from build123d import *

# Parameters (mm, degrees)
F0_R     = 4.1275
F0_R_2   = 4.0005
F0_W     = 107.95
F0_H     = 76.2
F0_R_3   = 3.429
F0_W_2   = 712.238387
F0_H_2   = 25.4
F0_W_3   = 19.05
F0_H_3   = 50.8
F1_DEPTH = 1.5748
F2_W     = 19.05
F2_H     = 1.5748
F3_DEPTH = 25.4


with BuildPart() as f1:
    # F0 (on Front) → F1 (new body)
    with BuildSketch(Plane.XZ):
        with BuildLine():
            Line((0, 71.12), (0, 0))
            Line((0, 0), (152.4, 0))
            Line((152.4, 0), (864.638387, 0))
            ThreePointArc((864.638387, 0), (866.755792, 0.026154), (868.871905, 0.1046))
            ThreePointArc((868.871905, 0.1046), (878.359069, 1.105153), (887.676316, 3.15364))
            ThreePointArc((887.676316, 3.15364), (903.696678, 9.414938), (918.144584, 18.748418))
            ThreePointArc((918.144584, 18.748418), (921.788387, 21.829358), (925.255116, 25.108271))
            Line((925.255116, 25.108271), (873.880221, 76.483166))
            ThreePointArc((873.880221, 76.483166), (871.544457, 74.285755), (868.777424, 72.664665))
            Line((868.777424, 72.664665), (830.221387, 55.5625))
            Line((830.221387, 55.5625), (830.221387, 36.5125))
            Line((830.221387, 36.5125), (747.671387, 36.5125))
            Line((747.671387, 36.5125), (747.671387, 112.7125))
            Line((747.671387, 112.7125), (830.221387, 112.7125))
            Line((830.221387, 112.7125), (830.221387, 100.0125))
            Line((830.221387, 100.0125), (862.984297, 100.0125))
            ThreePointArc((862.984297, 100.0125), (868.988044, 98.689863), (873.880221, 94.966834))
            Line((873.880221, 94.966834), (925.255116, 146.341729))
            ThreePointArc((925.255116, 146.341729), (921.788387, 149.620642), (918.144584, 152.701582))
            ThreePointArc((918.144584, 152.701582), (901.799905, 162.976519), (883.570429, 169.333333))
            ThreePointArc((883.570429, 169.333333), (874.163387, 170.91919), (864.638387, 171.45))
            Line((864.638387, 171.45), (858.288387, 171.45))
            Line((858.288387, 171.45), (839.238387, 171.45))
            Line((839.238387, 171.45), (839.238387, 222.25))
            Line((839.238387, 222.25), (839.238387, 273.05))
            Line((839.238387, 273.05), (839.238387, 323.85))
            Line((839.238387, 323.85), (595.3125, 200.025))
            Line((595.3125, 200.025), (455.231453, 200.025))
            Line((455.231453, 200.025), (439.727616, 200.025))
            Line((439.727616, 200.025), (356.5525, 200.025))
            Line((356.5525, 200.025), (356.5525, 151.765))
            Line((356.5525, 151.765), (303.2125, 151.765))
            Line((303.2125, 151.765), (303.2125, 200.025))
            Line((303.2125, 200.025), (71.490397, 200.025))
            Line((71.490397, 200.025), (0, 158.75))
            Line((0, 158.75), (0, 106.045))
            Line((0, 106.045), (138.1125, 106.045))
            ThreePointArc((138.1125, 106.045), (155.575, 88.5825), (138.1125, 71.12))
            Line((138.1125, 71.12), (0, 71.12))
        make_face()
        with Locations((184.0865, 65.0875)):
            Circle(F0_R, mode=Mode.SUBTRACT)
        Polygon((206.375, 41.91), (206.375, 88.5825), (206.375, 111.76), (266.7, 111.76), (266.7, 41.91), align=None, mode=Mode.SUBTRACT)
        with Locations((31.0642, 136.9695)):
            Circle(F0_R_2, mode=Mode.SUBTRACT)
        with Locations((184.0865, 109.8169)):
            Circle(F0_R, mode=Mode.SUBTRACT)
        with Locations((227.838, 136.9695)):
            Circle(F0_R_2, mode=Mode.SUBTRACT)
        with Locations((424.6118, 136.9695)):
            Circle(F0_R_2, mode=Mode.SUBTRACT)
        with BuildLine():
            ThreePointArc((853.652887, 31.8135), (848.509387, 36.957), (853.652887, 42.1005))
            Line((853.652887, 42.1005), (863.939887, 42.1005))
            ThreePointArc((863.939887, 42.1005), (867.576891, 40.594004), (869.083387, 36.957))
            ThreePointArc((869.083387, 36.957), (867.576891, 33.319996), (863.939887, 31.8135))
            Line((863.939887, 31.8135), (853.652887, 31.8135))
        make_face(mode=Mode.SUBTRACT)
        with Locations((642.388387, 74.6252)):
            Rectangle(F0_W, F0_H, mode=Mode.SUBTRACT)
        with BuildLine():
            ThreePointArc((715.794387, 106.0577), (719.921887, 110.1852), (724.049387, 106.0577))
            Line((724.049387, 106.0577), (724.049387, 47.6377))
            ThreePointArc((724.049387, 47.6377), (719.921887, 43.5102), (715.794387, 47.6377))
            Line((715.794387, 47.6377), (715.794387, 106.0577))
        make_face(mode=Mode.SUBTRACT)
        with Locations((621.3856, 136.9695)):
            Circle(F0_R_2, mode=Mode.SUBTRACT)
        with Locations((816.314887, 137.033)):
            Circle(F0_R_2, mode=Mode.SUBTRACT)
        with BuildLine():
            ThreePointArc((853.652887, 129.2225), (848.509387, 134.366), (853.652887, 139.5095))
            Line((853.652887, 139.5095), (863.939887, 139.5095))
            ThreePointArc((863.939887, 139.5095), (867.576891, 138.003004), (869.083387, 134.366))
            ThreePointArc((869.083387, 134.366), (867.576891, 130.728996), (863.939887, 129.2225))
            Line((863.939887, 129.2225), (853.652887, 129.2225))
        make_face(mode=Mode.SUBTRACT)
        with BuildLine():
            ThreePointArc((244.6655, 177.038), (247.988195, 175.661695), (249.3645, 172.339))
            ThreePointArc((249.3645, 172.339), (247.988195, 169.016305), (244.6655, 167.64))
            Line((244.6655, 167.64), (235.2675, 167.64))
            ThreePointArc((235.2675, 167.64), (230.5685, 172.339), (235.2675, 177.038))
            Line((235.2675, 177.038), (244.6655, 177.038))
        make_face(mode=Mode.SUBTRACT)
        with Locations((371.7925, 190.119)):
            Circle(F0_R_3, mode=Mode.SUBTRACT)
        with Locations((757.513887, 160.655)):
            Circle(F0_R_2, mode=Mode.SUBTRACT)
        with Locations((807.577287, 160.655)):
            Circle(F0_R_2, mode=Mode.SUBTRACT)
        with BuildLine():
            ThreePointArc((873.880221, 94.966834), (876.39713, 90.647253), (877.271797, 85.725))
            Line((877.271797, 85.725), (950.363387, 85.725))
            ThreePointArc((950.363387, 85.725), (950.230582, 90.49489), (949.832577, 95.25))
            ThreePointArc((949.832577, 95.25), (943.83796, 118.530537), (931.614968, 139.231197))
            ThreePointArc((931.614968, 139.231197), (928.534029, 142.875), (925.255116, 146.341729))
            Line((925.255116, 146.341729), (873.880221, 94.966834))
        make_face()
        with BuildLine():
            Line((873.880221, 76.483166), (925.255116, 25.108271))
            ThreePointArc((925.255116, 25.108271), (928.534029, 28.575), (931.614968, 32.218803))
            ThreePointArc((931.614968, 32.218803), (943.83796, 52.919463), (949.832577, 76.2))
            ThreePointArc((949.832577, 76.2), (950.230582, 80.95511), (950.363387, 85.725))
            Line((950.363387, 85.725), (877.271797, 85.725))
            ThreePointArc((877.271797, 85.725), (876.39713, 80.802747), (873.880221, 76.483166))
        make_face()
        with BuildLine():
            ThreePointArc((950.363387, 85.725), (950.230582, 80.95511), (949.832577, 76.2))
            Line((949.832577, 76.2), (962.601416, 76.2))
            ThreePointArc((962.601416, 76.2), (962.947826, 80.956902), (963.063387, 85.725))
            Line((963.063387, 85.725), (950.363387, 85.725))
        make_face()
        with BuildLine():
            ThreePointArc((949.832577, 95.25), (950.230582, 90.49489), (950.363387, 85.725))
            Line((950.363387, 85.725), (963.063387, 85.725))
            Line((963.063387, 85.725), (962.601416, 95.25))
            Line((962.601416, 95.25), (949.832577, 95.25))
        make_face()
        with BuildLine():
            Line((934.235372, 155.321985), (925.255116, 146.341729))
            ThreePointArc((925.255116, 146.341729), (928.534029, 142.875), (931.614968, 139.231197))
            Line((931.614968, 139.231197), (940.643901, 148.26013))
            ThreePointArc((940.643901, 148.26013), (937.525213, 151.868717), (934.235372, 155.321985))
        make_face()
        with BuildLine():
            ThreePointArc((918.144584, 152.701582), (921.788387, 149.620642), (925.255116, 146.341729))
            Line((925.255116, 146.341729), (934.235372, 155.321985))
            ThreePointArc((934.235372, 155.321985), (930.782104, 158.611826), (927.173517, 161.730514))
            Line((927.173517, 161.730514), (918.144584, 152.701582))
        make_face()
        with BuildLine():
            ThreePointArc((864.638387, 171.45), (874.163387, 170.91919), (883.570429, 169.333333))
            Line((883.570429, 169.333333), (883.598973, 182.306452))
            ThreePointArc((883.598973, 182.306452), (874.163387, 183.688029), (864.638387, 184.15))
            Line((864.638387, 184.15), (864.638387, 171.45))
        make_face()
        with BuildLine():
            ThreePointArc((931.614968, 32.218803), (928.534029, 28.575), (925.255116, 25.108271))
            Line((925.255116, 25.108271), (934.235372, 16.128015))
            ThreePointArc((934.235372, 16.128015), (937.525213, 19.581283), (940.643901, 23.18987))
            Line((940.643901, 23.18987), (931.614968, 32.218803))
        make_face()
        with BuildLine():
            ThreePointArc((925.255116, 25.108271), (921.788387, 21.829358), (918.144584, 18.748418))
            Line((918.144584, 18.748418), (927.173517, 9.719486))
            ThreePointArc((927.173517, 9.719486), (930.782104, 12.838174), (934.235372, 16.128015))
            Line((934.235372, 16.128015), (925.255116, 25.108271))
        make_face()
        with BuildLine():
            ThreePointArc((887.676316, 3.15364), (878.359069, 1.105153), (868.871905, 0.1046))
            Line((868.871905, 0.1046), (868.871905, -12.60891))
            ThreePointArc((868.871905, -12.60891), (878.368219, -11.737671), (887.735648, -9.951524))
            Line((887.735648, -9.951524), (887.676316, 3.15364))
        make_face()
        with Locations((508.519193, -12.7)):
            Rectangle(F0_W_2, F0_H_2)
        with Locations((848.763387, 196.85)):
            Rectangle(F0_W_3, F0_H_3)
        with Locations((848.763387, 298.45)):
            Rectangle(F0_W_3, F0_H_3)
        Polygon((356.5525, 212.725), (356.5525, 200.025), (439.727616, 200.025), (455.231453, 200.025), (595.3125, 200.025), (579.161286, 212.725), align=None)
        Polygon((95.536456, 212.725), (71.490397, 200.025), (303.2125, 200.025), (303.2125, 212.725), align=None)
        Polygon((0, 173.414697), (0, 158.75), (71.490397, 200.025), (57.889698, 206.837329), align=None)
    extrude(amount=F1_DEPTH)

    # F2 (on face) → F3 (cut)
    with BuildSketch(Plane.XZ.offset(1.5748)):
        with Locations((848.763387, 172.2374)):
            Rectangle(F2_W, F2_H)
    extrude(amount=-F3_DEPTH, mode=Mode.SUBTRACT)


solid = f1.part
Work out the finished part from the listing and answer in its coordinate system (mm). A direction names the side the tool comes from. Round coordinates to 2 decimals unless told otherwise and drop trailing zeros. Loops run counter-clockwise (first coordinate to the right, second up) from the corner with the lowest first, then second, coordinate; pieces in that order, holes last. Notation, with made-up numbers: (82.25, -25) -> (103.25, -25) arc R16 cw to (103.25, -21) -> close; hole circle Ø9 at (-13.5, 15.5). An arc over 180 degrees is marked (long way). Use one line per item in the form item = value.
(1) A tool of negligible diameter and unlimited length cuts with its end or side. For faces 1 (the cylindrical face through (943.967, -0.776, 118.218)), 2 (the cylindrical face through (155.57, -0.78, 88.97)), 3 (the flat face through (849.769, -0.776, 64.233)), from which of +Z, -Z, +X, -X, +Y, -Y can it reach the whole face along a straight path? Write none if from no direction.
Answer list:
face_1 = +X, +Y, -Y
face_2 = -X, +Y, -Y
face_3 = +Y, -Y
(2) For a pull along X with two mould halves and no side action, classify faces 4 (the flat face through (29.35, -0.78, 190.36)), 5 (the cylindrical face through (903.482, -0.776, 9.305)), 6 (the flat face through (475, 0, 113)), 7 (the cylindrical face through (902.04, -0.78, 162.86)) as released by +X, released by -X, zero draft, split by the parting line, or undercut.
Answer list:
face_4 = released by -X
face_5 = undercut
face_6 = zero draft
face_7 = undercut
(3) Straight lines are drawn through the part: line 1 (X direction, y = -0.65, z = 201); line 2 (Z direction, x = 249.5, y = -1.15) (3 decimals); line 3 (X direction, y = -0.8, z = 179.5). For each, find the intervals that lie inside material, in ascending order.
Answer list:
line_1 = 47.78 to 69.54, 73.34 to 303.21, 356.55 to 594.07, 597.23 to 858.29
line_2 = -25.4 to 41.91, 111.76 to 212.725
line_3 = 10.54 to 303.21, 356.55 to 858.29, 864.64 to 883.59
(4) Find section D-D on z = 301.5. Give the vertices of the cut face in (x, y), then the cut area to 3 significant figures.
Answer list:
outline = (795.21, -1.57) -> (858.29, -1.57) -> (858.29, 0) -> (795.21, 0) -> close
area = 99.3 mm2
(5) Find section B-B on y = -1.3. Give the number of separate pieces and of enclosed holes in the cut face, then the cut area to 3 significant figures.
Answer list:
separate_pieces = 1
enclosed_holes = 17
area = 196,000 mm2
(6) Find section C-C on z = 253.5. Give the vertices of the cut face in (x, y).
Answer list:
outline = (700.65, -1.57) -> (839.24, -1.57) -> (839.24, 0) -> (700.65, 0) -> close
(7) Flat-ended cylindrical pins translate along their axes: P1, Ø0.8, axis at x = 335, y = -0.5, coming from the +Z side (3 decimals); P2, Ø0.5, axis at y = -0.5, z = 62.5, coming from the -X side. Find the tip coordinate at first contact, or state that the pin passes through.
Answer list:
P1 = 151.765
P2 = 0
(8) Find section A-A on x = 773. Give the vertices of the cut face in (y, z).
Answer list:
outline = (-1.57, -25.4) -> (0, -25.4) -> (0, 36.51) -> (-1.57, 36.51) -> close; (-1.57, 112.71) -> (0, 112.71) -> (0, 290.23) -> (-1.57, 290.23) -> close
